from build123d import *

# Parameters (mm, degrees)
BOSS_EXTRUDE1_DEPTH     = 47.75
SHELL2_T                = -1.2
SKETCH2_W               = 45.35
SKETCH2_H               = 17.927015757
CUT_EXTRUDE1_DEPTH      = 57.531559043
CUT_EXTRUDE2_DEPTH      = 58.038533691
CUT_EXTRUDE2_DEPTH_BACK = 58.038533691
BOSS_EXTRUDE2_DEPTH     = 3.5
CUT_EXTRUDE3_DEPTH      = 58.038533691
SKETCH7_R               = 2.45
SKETCH7_R_2             = 1.35
BOSS_EXTRUDE3_DEPTH     = 1.8
SHELL3_START            = -46.25
SHELL3_DEPTH            = 44.75
SHELL3_2_OUTLINE_W      = 2
SHELL3_2_OUTLINE_H      = 16.790482419
SHELL3_2_DEPTH          = 4.8
SHELL3_START_2          = -6.3
SHELL3_3_OUTLINE_W      = 2
SHELL3_3_OUTLINE_H      = 16.790482419
SHELL3_3_DEPTH          = 4.8
SKETCH8_R               = 1.5
SKETCH8_R_2             = 0.7
BOSS_EXTRUDE4_DEPTH     = 1.8
FILLET1_R               = 3.5


# Read off the part's stored shape, not the designer's step: Shell3
with BuildPart() as part:
    # Sketch1 → Boss-Extrude1 (new body)
    with BuildSketch(Plane(origin=(0, 0, 0), x_dir=(0, 0, -1), z_dir=(1, 0, 0))):
        Polygon((0, 0), (0, 19.2), (-7.46, 19.2), (-24.590482419, 0), align=None)
    extrude(amount=-BOSS_EXTRUDE1_DEPTH)

    # Shell2
    shell2_openings = [part.faces().sort_by_distance(p)[0] for p in [
        (-23.875, 0, 12.29524121),
    ]]
    offset(amount=SHELL2_T, openings=shell2_openings, kind=Kind.INTERSECTION)

    # Sketch2 → Cut-Extrude1 (cut, through all)
    with BuildSketch(Plane.XY.offset(1.2)):
        with Locations((-23.875, 8.963507878)):
            Rectangle(SKETCH2_W, SKETCH2_H)
    extrude(amount=-CUT_EXTRUDE1_DEPTH, mode=Mode.SUBTRACT)

    # Sketch3 → Cut-Extrude2 (cut, two sides: drawn at the far end of the back side and taken through both)
    with BuildSketch(Plane(origin=(0, 19.2, 0), x_dir=(1, 0, 0), z_dir=(0, 1, 0)).offset(-CUT_EXTRUDE2_DEPTH_BACK)):
        Polygon((-41.25, 106.046953634), (-41.25, 0), (-41.25, -5.96), (-6.5, -5.96), (-6.5, 0), (-6.5, 106.046953634), (-6.5, 318.140860903), (-41.25, 318.140860903), align=None)
    extrude(amount=CUT_EXTRUDE2_DEPTH + CUT_EXTRUDE2_DEPTH_BACK, mode=Mode.SUBTRACT)

    # Sketch5 → Boss-Extrude2 (add)
    with BuildSketch(Plane.XZ):
        Polygon((-47.75, 0), (-39.95, 0), (-39.95, 16.790482419), (-7.8, 16.790482419), (-7.8, 0), (0, 0), (0, 24.590482419), (-47.75, 24.590482419), align=None)
    extrude(amount=-BOSS_EXTRUDE2_DEPTH)

    # Sketch6 → Cut-Extrude3 (cut, through all)
    with BuildSketch(Plane.ZY.offset(47.75)):
        Polygon((21.467738228, 3.5), (24.590482419, 0), (24.590482419, 3.5), align=None)
    extrude(amount=-CUT_EXTRUDE3_DEPTH, mode=Mode.SUBTRACT)

    # Sketch7 → Boss-Extrude3 (add)
    # profile 1 of 2: a face of its own
    with BuildSketch(Plane(origin=(0, 19.2, 0), x_dir=(1, 0, 0), z_dir=(0, 1, 0))):
        with Locations(Location((-44.5, -3.73, 0), (0, 0, 270))):
            Circle(SKETCH7_R)
        with Locations(Location((-44.5, -3.73, 0), (0, 0, 270))):
            Circle(SKETCH7_R_2, mode=Mode.SUBTRACT)
    # profile 2 of 2: a face of its own
    with BuildSketch(Plane(origin=(0, 19.2, 0), x_dir=(1, 0, 0), z_dir=(0, 1, 0))):
        with Locations(Location((-3.25, -3.73, 0), (0, 0, 270))):
            Circle(SKETCH7_R)
        with Locations(Location((-3.25, -3.73, 0), (0, 0, 270))):
            Circle(SKETCH7_R_2, mode=Mode.SUBTRACT)
    extrude(amount=BOSS_EXTRUDE3_DEPTH)

    # Shell3 outline → Shell3 (cut)
    with BuildSketch(Plane.YZ.offset(SHELL3_START)):
        Polygon((2, 18.290482419), (2, 20.795809028), (0, 22.58023428), (0, 18.290482419), align=None)
    extrude(amount=SHELL3_DEPTH, mode=Mode.SUBTRACT)

    # Shell3 2 outline → Shell3 2 (cut)
    with BuildSketch(Plane.YZ.offset(SHELL3_START)):
        with Locations((1, 9.895241209)):
            Rectangle(SHELL3_2_OUTLINE_W, SHELL3_2_OUTLINE_H)
    extrude(amount=SHELL3_2_DEPTH, mode=Mode.SUBTRACT)

    # Shell3 3 outline → Shell3 3 (cut)
    with BuildSketch(Plane.YZ.offset(SHELL3_START_2)):
        with Locations((1, 9.895241209)):
            Rectangle(SHELL3_3_OUTLINE_W, SHELL3_3_OUTLINE_H)
    extrude(amount=SHELL3_3_DEPTH, mode=Mode.SUBTRACT)

    # Sketch8 → Boss-Extrude4 (add)
    # profile 1 of 4: a face of its own
    with BuildSketch(Plane.XZ.offset(-2)):
        with Locations(Location((-43.85, 8.196666667, 0), (0, 0, 270))):
            Circle(SKETCH8_R)
        with Locations(Location((-43.85, 8.196666667, 0), (0, 0, 270))):
            Circle(SKETCH8_R_2, mode=Mode.SUBTRACT)
    # profile 2 of 4: a face of its own
    with BuildSketch(Plane.XZ.offset(-2)):
        with Locations(Location((-43.85, 16.393333333, 0), (0, 0, 270))):
            Circle(SKETCH8_R)
        with Locations(Location((-43.85, 16.393333333, 0), (0, 0, 270))):
            Circle(SKETCH8_R_2, mode=Mode.SUBTRACT)
    # profile 3 of 4: a face of its own
    with BuildSketch(Plane.XZ.offset(-2)):
        with Locations(Location((-3.9, 16.393333333, 0), (0, 0, 90))):
            Circle(SKETCH8_R)
        with Locations(Location((-3.9, 16.393333333, 0), (0, 0, 270))):
            Circle(SKETCH8_R_2, mode=Mode.SUBTRACT)
    # profile 4 of 4: a face of its own
    with BuildSketch(Plane.XZ.offset(-2)):
        with Locations(Location((-3.9, 8.196666667, 0), (0, 0, 90))):
            Circle(SKETCH8_R)
        with Locations(Location((-3.9, 8.196666667, 0), (0, 0, 270))):
            Circle(SKETCH8_R_2, mode=Mode.SUBTRACT)
    extrude(amount=BOSS_EXTRUDE4_DEPTH)

    # Fillet1
    fillet1_edges = [part.edges().sort_by_distance(p)[0] for p in [
        (-47.75, 9.6, 16.02524121),
        (0, 9.6, 16.02524121),
        (-41.25, 18.563507879, 0),
        (-6.5, 18.563507879, 0),
    ]]
    fillet(fillet1_edges, radius=FILLET1_R)


solid = part.part
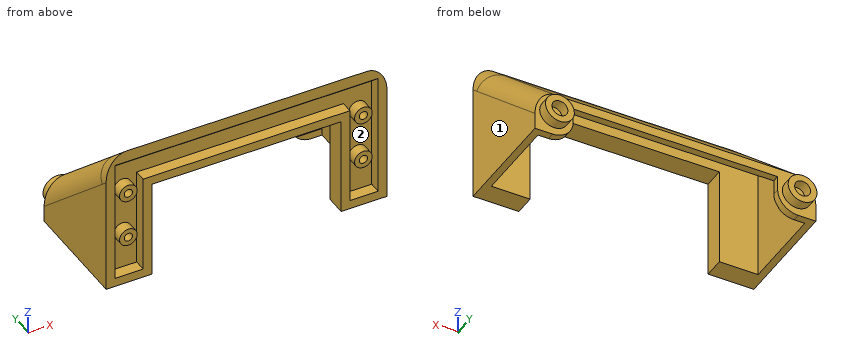
Build history of the part. All positions in model axes, mm. Face numbers are marked on the shaded views. Coordinates: 2 decimals unless noted, no trailing zeros. Write each loop counter-clockwise with the first axis right and the second up, starting at its lowest first coordinate (ties: lowest second). Pieces come first, ordered by that corner, then holes. Notation, with made-up numbers: (87.25, 72.25) -> (134.25, 72.25) arc R27 cw to (134.25, 95.25) -> close; hole circle Ø5 at (-17, 34.25). An arc over 180 degrees is marked (long way). Use CSV: the item, a comma, the result in double quotes. Start each with the question number.
Q1. Drill centre lines: probe 1 along Y at (x, z) = (-43.5, 6.5); probe 2 along X at (y, z) = (13.75, 6.5); probe 3 along Y at (x, z) = (-41, 13). Where is each one in solid material? Low to high.
Q2. Pull direction Z, two halves, no side cores. Call the marked faces 1 and 2: released by +Z, released by -Z, zero draft, split by the parting line, or undercut.
Q3. Flat gauge pins, fed straight in: pin 1 Ø2 at (x, y) = (-33, 17.5) entering from -Z; pin 2 Ø1.5 at (x, z) = (-44, 8.5) entering from -Y; pin 3 Ø3 at (x, y) = (-38, 2.5) entering from -Z. Where does each tip first touch, or does it go through?
Q4. Cut at A-A, the plane x = -13.5. List the corners of the cut face in (y, z), then the cut area to 3 significant figures.
Checked values:
1,probe 1,"y = 2 to 3.5, 18 to 19.2"
1,probe 2,"x = -47.75 to -46.55, -1.2 to 0"
1,probe 3,"y = 0 to 3.5, 11.19 to 12.99"
2,face 1,"zero draft"
2,face 2,"undercut"
3,pin 1,"stops at z = 5.96"
3,pin 2,"stops at y = 0.2"
3,pin 3,"stops at z = 16.79"
4,outline,"(0, 16.79) -> (3.5, 16.79) -> (3.5, 19.86) -> (18, 6.92) -> (18, 5.96) -> (19.2, 5.96) -> (19.2, 7.46) -> (0, 24.59) -> (0, 22.58) -> (2, 20.8) -> (2, 18.29) -> (0, 18.29) -> close"
4,area,"40.8 mm²"
